Autodesk Fusion 360 part; units mm, degrees
cylinder "CylinderPrimitive1" add diameter 40 height 5 placed x (1, 0, 0) y (0, 1, 0) z (0, 0, 1) at (0, 0, 0)
hole "Hole1" at (0, 0, 5) direction (0, 0, -1) diameter 20.5 depth 3.75 tip angle 180
fillet "Fillet1" radius 1 1 edges at (-18.6465, 7.2323, 0)
Input: part model. Units: mm. Frame: model coordinates. A direction names the side the tool comes from. Give positions to 0.01 mm unless a question says otherwise; leave off trailing zeros. Write each loop counter-clockwise with the first axis right and the second up, starting at its lowest first coordinate (ties: lowest second). Pieces come first, ordered by that corner, then holes. Notation, with made-up numbers: M 47,-15 L 106,-15 A17 cw 106,15 Z; hole C 34.25,-33 d11. An arc over 180 degrees is marked long. Write item = value, one per line. Start each with the question number.
1) Cut plane C-C on z = 4.05. Return the cut outline in (x, y), then the cut area to 3 significant figures.
2) First-contact query: pin 1 Ø10 at (x, y) = (7.5, 14) entering from -Z; pin 2 Ø1 at (x, z) = (-1.5, 2) entering from +Y (3 decimals); pin 3 Ø2 at (y, z) = (-4.5, 1) entering from -X; pin 4 Ø2 at (x, y) = (-8.5, 2) entering from +Z. Flat tips, straight axial feed; report the tip coordinate or a pass-through.
3) Material intervals for line 1 along Y through (x, z) = (0, 3.4); line 2 along Z through (x, y) = (-1.5, -7.5); line 3 along X through (y, z) = (-8.5, 4.75), sorted ascending. Write a range as [from, to].
4) Reachability of faces 1 (the cylindrical face through (10.006, 2.222, 3.099)), 2 (the flat face through (9, -9, 5)) from +Z, -Z, +X, -X, +Y, -Y: full face, straight path, thin tool, end or side. Return the list, or none.
5) Cut plane A-A on x = 0. Return the cut outline in (y, z), then the cut area to 3 significant figures.
6) Draft query along X for faces 3 (the cylindrical face through (-4.336, -19.524, 3.028)), 4 (the flat face through (0, 0, 0)), 5 (the flat face through (0, 0, 1.25)). Return one class per face: +X half, -X half, draft (parallel to the pull), parting line (faces both ways), or undercut.
Solved:
q1.outline = C 0,0 d40; hole C 0,0 d20.5
q1.area = 927 mm2
q2.pin_1 = 0
q2.pin_2 = 19.975
q2.pin_3 = -19.69
q2.pin_4 = 1.25
q3.line_1 = [-20, -10.25], [10.25, 20]
q3.line_2 = [0, 1.25]
q3.line_3 = [-18.1, -5.73], [5.73, 18.1]
q4.face_1 = +Z
q4.face_2 = +Z, +X, -X, +Y, -Y
q5.outline = M -20,1 A1 ccw -19,0 L 19,0 A1 ccw 20,1 L 20,5 L 10.25,5 L 10.25,1.25 L -10.25,1.25 L -10.25,5 L -20,5 Z
q5.area = 123 mm2
q6.face_3 = parting line
q6.face_4 = draft
q6.face_5 = undercut
